from build123d import *

# Parameters (mm, degrees)
SKETCH1_R           = 14.1605
SKETCH1_R_2         = 2.38125
BOSS_EXTRUDE2_DEPTH = 3.175
SKETCH2_R           = 2.38125
CUT_EXTRUDE1_DEPTH  = 4.175
SKETCH3_R           = 2.38125
CUT_EXTRUDE2_DEPTH  = 3.175
SKETCH6_R           = 2.5527
CUT_EXTRUDE3_DEPTH  = 4.175


with BuildPart() as part:
    # Sketch1 → Boss-Extrude2 (new body)
    with BuildSketch(Plane.ZY.offset(-2085.27445945)):
        with BuildLine():
            Line((-676.476495312, -196.108668054), (-644.862434405, -195.889095816))
            ThreePointArc((-644.862434405, -195.889095816), (-640.385331878, -193.998083759), (-638.556689771, -189.495146754))
            Line((-638.556689771, -189.495146754), (-639.372580729, -72.022980064))
            ThreePointArc((-639.372580729, -72.022980064), (-637.543938621, -67.520043059), (-633.066836095, -65.629031002))
            Line((-633.066836095, -65.629031002), (-553.190076911, -65.074255113))
            ThreePointArc((-553.190076911, -65.074255113), (-549.514401488, -64.099885183), (-546.767272269, -61.470575839))
            Line((-546.767272269, -61.470575839), (-527.590173696, -30.548905962))
            ThreePointArc((-527.590173696, -30.548905962), (-524.819944777, -27.906688623), (-521.114446397, -26.945042905))
            Line((-521.114446397, -26.945042905), (-478.726560046, -26.945042905))
            ThreePointArc((-478.726560046, -26.945042905), (-475.067517944, -27.88104628), (-472.307393362, -30.459108288))
            Line((-472.307393362, -30.459108288), (-452.701509897, -61.110700599))
            ThreePointArc((-452.701509897, -61.110700599), (-450.356282883, -63.444285805), (-447.243078231, -64.563958281))
            ThreePointArc((-447.243078231, -64.563958281), (-442.043441328, -65.791181786), (-437.215518263, -68.078857532))
            ThreePointArc((-437.215518263, -68.078857532), (-394.361205687, -65.922698326), (-380.69060226, -25.250155611))
            Line((-380.69060226, -25.250155611), (-381.274246521, -23.172734147))
            ThreePointArc((-381.274246521, -23.172734147), (-381.931013294, -21.160982924), (-382.752967438, -19.210886269))
            Line((-382.752967438, -19.210886269), (-405.028313451, 28.035268168))
            ThreePointArc((-405.028313451, 28.035268168), (-408.719025679, 32.64446469), (-414.095120009, 35.086525107))
            Line((-414.095120009, 35.086525107), (-713.524757665, 93.219773114))
            ThreePointArc((-713.524757665, 93.219773114), (-714.988859477, 93.729040419), (-716.419168956, 94.326670824))
            ThreePointArc((-716.419168956, 94.326670824), (-737.189413392, 97.405032689), (-756.436338691, 89.012462628))
            Line((-756.436338691, 89.012462628), (-808.634266444, 45.900443365))
            ThreePointArc((-808.634266444, 45.900443365), (-815.475018373, 37.06060929), (-817.858650965, 26.140130862))
            Line((-817.858650965, 26.140130862), (-817.070267282, -87.371532031))
            ThreePointArc((-817.070267282, -87.371532031), (-809.568913511, -105.217897447), (-791.670879889, -112.595123175))
            Line((-791.670879889, -112.595123175), (-772.445079401, -112.595123175))
            ThreePointArc((-772.445079401, -112.595123175), (-738.471128747, -122.447936138), (-715.040138137, -148.948802642))
            Line((-715.040138137, -148.948802642), (-699.614880674, -181.567808874))
            ThreePointArc((-699.614880674, -181.567808874), (-690.167883624, -192.215217755), (-676.476495312, -196.108668054))
        make_face()
        with Locations((-732.173834383, 59.636607157)):
            Circle(SKETCH1_R, mode=Mode.SUBTRACT)
        with Locations((-779.099930223, -68.570323835)):
            Circle(SKETCH1_R, mode=Mode.SUBTRACT)
        with Locations((-654.585392145, -186.431395895)):
            Circle(SKETCH1_R_2, mode=Mode.SUBTRACT)
        with Locations((-629.958065992, -56.082209622)):
            Circle(SKETCH1_R_2, mode=Mode.SUBTRACT)
        with Locations((-553.895503221, -55.553924847)):
            Circle(SKETCH1_R_2, mode=Mode.SUBTRACT)
        with Locations((-417.370503221, -35.55524491)):
            Circle(SKETCH1_R, mode=Mode.SUBTRACT)
    extrude(amount=BOSS_EXTRUDE2_DEPTH)

    # Sketch2 → Cut-Extrude1 (cut, through all)
    with BuildSketch(Plane(origin=(2085.27445945, 0, 0), x_dir=(0, 0, -1), z_dir=(1, 0, 0))):
        with Locations((732.173834383, 85.036607157)):
            Circle(SKETCH2_R)
        with Locations((732.173834383, 34.236607157)):
            Circle(SKETCH2_R)
        with Locations((750.134264867, 41.676013157)):
            Circle(SKETCH2_R)
        with Locations((714.213403899, 77.597201157)):
            Circle(SKETCH2_R)
        with Locations((750.134264867, 77.597201157)):
            Circle(SKETCH2_R)
        with Locations((714.213403899, 41.676013157)):
            Circle(SKETCH2_R)
    extrude(amount=-CUT_EXTRUDE1_DEPTH, mode=Mode.SUBTRACT)

    # Sketch3 → Cut-Extrude2 (cut)
    with BuildSketch(Plane(origin=(2085.27445945, 0, 0), x_dir=(0, 0, -1), z_dir=(1, 0, 0))):
        with Locations((759.618090186, -100.982485439)):
            Circle(SKETCH3_R)
        with Locations((541.187693092, 46.53204311)):
            Circle(SKETCH3_R)
        with Locations((478.851639869, 34.42970992)):
            Circle(SKETCH3_R)
        with Locations((416.515586647, 22.327376731)):
            Circle(SKETCH3_R)
        with Locations((525.320503221, -14.245042905)):
            Circle(SKETCH3_R)
        with Locations((798.886947172, 37.479390763)):
            Circle(SKETCH3_R)
        with Locations((665.859799537, 70.736709489)):
            Circle(SKETCH3_R)
        with Locations((603.523746314, 58.634376299)):
            Circle(SKETCH3_R)
        with Locations((703.559149884, -143.519538535)):
            Circle(SKETCH3_R)
        with Locations((726.384244699, -115.392244277)):
            Circle(SKETCH3_R)
        with Locations((804.898658391, -11.249556635)):
            Circle(SKETCH3_R)
        with Locations((474.520503221, -14.245042905)):
            Circle(SKETCH3_R)
        with Locations((651.589984927, -141.551336746)):
            Circle(SKETCH3_R)
        with Locations((651.589984927, -90.751336746)):
            Circle(SKETCH3_R)
        with Locations((593.128456503, -52.651336746)):
            Circle(SKETCH3_R)
    extrude(amount=-CUT_EXTRUDE2_DEPTH, mode=Mode.SUBTRACT)

    # Sketch6 → Cut-Extrude3 (cut, through all)
    with BuildSketch(Plane(origin=(2085.27445945, 0, 0), x_dir=(0, 0, -1), z_dir=(1, 0, 0))):
        with Locations((395.373457966, -48.25524491)):
            Circle(SKETCH6_R)
        with Locations((405.464253222, -56.177474837)):
            Circle(SKETCH6_R)
        with Locations((395.373457966, -22.85524491)):
            Circle(SKETCH6_R)
        with Locations((393.558003223, -35.55524491)):
            Circle(SKETCH6_R)
        with Locations((417.370503221, -10.15524491)):
            Circle(SKETCH6_R)
        with Locations((405.464253222, -14.933014983)):
            Circle(SKETCH6_R)
        with Locations((439.367548477, -22.85524491)):
            Circle(SKETCH6_R)
        with Locations((429.276753221, -14.933014983)):
            Circle(SKETCH6_R)
        with Locations((439.367548477, -48.25524491)):
            Circle(SKETCH6_R)
        with Locations((441.18300322, -35.55524491)):
            Circle(SKETCH6_R)
        with Locations((417.370503221, -60.95524491)):
            Circle(SKETCH6_R)
        with Locations((429.276753221, -56.177474837)):
            Circle(SKETCH6_R)
    extrude(amount=-CUT_EXTRUDE3_DEPTH, mode=Mode.SUBTRACT)


solid = part.part
Geometry: final body of the model. Coordinates: model frame, mm. A direction names the side the tool comes from. Give positions to 0.01 mm unless a question says otherwise; leave off trailing zeros. Write each loop counter-clockwise with the first axis right and the second up, starting at its lowest first coordinate (ties: lowest second). Pieces come first, ordered by that corner, then holes. Notation, with made-up numbers: (-5.5, -40) -> (9.5, -40) arc R20 ccw to (9.5, -33) -> close; hole circle Ø1 at (62.5, -7). An arc over 180 degrees is marked (long way). Answer as a JSON object with one key per item and string values.
1. Contact query for a flat-ended pin moving along its axis: pin 1 (1 mm diameter, centred on x = 2084, z = -495.5, fed in from -Y). Output: stop coordinate, or through.
Ans:
{"pin 1": "stops at y = -26.95"}
2. Cut plane C-C on z = -496.5. Output: boundary loops of the cut face in (x, y).
Ans:
{"outline": "(2082.1, -26.95) -> (2085.27, -26.95) -> (2085.27, 51.09) -> (2082.1, 51.09) -> close"}
3. Cut plane A-A on y = -78. Output: boundary loops of the cut face in (x, z), and give its area (3 significant figures).
Ans:
{"outline": "(2082.1, -817.14) -> (2085.27, -817.14) -> (2085.27, -789.66) -> (2082.1, -789.66) -> close; (2082.1, -768.54) -> (2085.27, -768.54) -> (2085.27, -639.33) -> (2082.1, -639.33) -> close", "area": "497 mm^2"}
4. Ray query, probe 1 along Y at (x, z) = (2084.8, -728); probe 2 along Z at (x, y) = (2084.3, -32); probe 3 along Z at (x, y) = (2083.7, 34). Return the intervals inside material, ascending. Write a range as from..to.
Ans:
{"probe 1": "y = -130.74..-117.14, -113.64..46.11, 73.17..97.51", "probe 2": "z = -817.45..-528.49, -471.32..-431.08, -403.66..-379.44", "probe 3": "z = -816.67..-734.54, -729.8..-481.19, -476.51..-410.88"}
5. Cut plane B-B on x = 2084.25. Count the separate pieces of the cut face and the enclosed holes in it, and give its area (3 significant figures).
Ans:
{"separate pieces": "1", "enclosed holes": "39", "area": "65,500 mm^2"}
6. Cut plane D-D on y = -173. Output: boundary loops of the cut face in (x, z), and give its area (3 significant figures).
Ans:
{"outline": "(2082.1, -703.67) -> (2085.27, -703.67) -> (2085.27, -638.67) -> (2082.1, -638.67) -> close", "area": "206 mm^2"}
7. Access query for faces 5 (the cylindrical face through (2083.709, 97.443, -736.894)), 6 (the flat face through (2083.71, -45.57, -462.64)). Directions: +Z, -Z, +X, -X, +Y, -Y. A direction counts if a zero-diameter tool reaches every point of the face in a straight line with its end or side. Return the directions, or none.
Ans:
{"face 5": "+X, -X, +Y", "face 6": "+X, -X, -Y"}
8. Mould query, pull axis Z, two halves, no side actions, for faces 1 (the flat face through (2083.709, -46.226, -537.313)), 2 (the flat face through (2082.099, -14, -650)), 3 (the flat face through (2083.709, 4.081, -393.735)), 4 (the cylindrical face through (2083.71, -122.18, -738.9)). Classes: pulls with the +Z half, pulls with the -Z half, needs draft (parallel to the pull), parting line crosses it, or undercut.
Ans:
{"face 1": "undercut", "face 2": "needs draft", "face 3": "pulls with the +Z half", "face 4": "pulls with the -Z half"}
